Design review of the part built by this model. Coordinates are the model's own, in mm. A direction names the side the tool comes from. Coordinates: 2 decimals unless noted, no trailing zeros. Loops run counter-clockwise (first coordinate to the right, second up) from the corner with the lowest first, then second, coordinate; pieces in that order, holes last. Notation, with made-up numbers: (-39.5, 10.5) - (-2.5, 10.5) arc R21 cw to (-2.5, 30.5) - close; hole circle Ø8 at (-1.75, 71.25). An arc over 180 degrees is marked (long way). Answer in a Markdown table with one row per item. Add a question column.
(1) Clearance check with flat-ended pins moving along their axes: pin 1 (12 mm diameter, centred on y = 14, z = -4.5, fed in from -X); pin 2 (5 mm diameter, centred on y = 18, z = -3.5, fed in from +X); pin 3 (0.8 mm diameter, centred on x = -7, z = 0.5, fed in from +Y); pin 4 (3 mm diameter, centred on y = 14, z = -2, fed in from +X). State where each tip first meets the part, or that it passes through.
(2) We need section B-B, the plane x = 0. Write out the cut boundary in (y, z), plus the area to 3 significant figures.
(3) The part is to be moulded in two halves that separate along X. For faces 1 (the face through (3.3, 21.9, -0.1)), 2 (the face through (-8.321, 13.492, 0.845)), 3 (the face through (0.07, 37.76, 2.64)), say which applies: released by +X, released by -X, zero draft, split by the parting line, or undercut.
(4) We need section C-C, the plane y = 8.5. Write out the cut boundary in (x, z).
(5) We need section D-D, the plane y = 14.5. Write out the cut boundary in (x, z).
(6) For faces 4 (the face through (0, 37.9, 0)), 5 (the face through (0, 32, -1)), 6 (the face through (-1.08, 17.34, -4.88)), 7 (the face through (-7, 14.1, 0)), list the 3-axis set-ups (+Z, -Z, +X, -X, +Y, -Y) from which the entire face can be reached by the end or side of a thin tool; tool diameter is ignored.
(7) We need section A-A, the plane z = 0. Write out the cut boundary in (x, y).
(8) To check wall thickness, follow L1, parallel to Y at x = 0.5, z = 10; L2, parallel to X at y = 27, z = 0; L3, parallel to X at y = 22, z = -1. State the ranges of each line that lie inside material, in increasing order. Write a range as [from, to].
Autodesk Inventor part; units mm, degrees
ref_plane "YZ Plane" through (0, 0, 0) normal (1, 0, 0) x (0, 1, 0)
ref_plane "XZ Plane" through (0, 0, 0) normal (0, 1, 0) x (-1, 0, 0)
ref_plane "XY Plane" through (0, 0, 0) normal (0, 0, 1) x (1, 0, 0)
sketch "Sketch1" plane through (0, 0, 0) normal (0, 1, 0) x (-1, 0, 0)
  circle A0 centre (0, 0) radius 11.1
  dimension "d0" = 22.2
extrude "Extrusion1" add sketch "Sketch1" along normal blind 12.9
fillet "Fillet1" radius 0.3 1 edges at (11.1, 12.9, 0)
sketch "Sketch2" plane through (0, 12.9, 0) normal (0, 1, 0) x (1, 0, 0)
  circle A0 centre (0, 0) radius 5
  dimension "d4" = 10
extrude "Extrusion2" add sketch "Sketch2" along normal blind 9
sketch "Sketch3" plane through (0, 21.9, 0) normal (0, 1, 0) x (1, 0, 0)
  circle A0 centre (0, 0) radius 3
  dimension "d9" = 6
extrude "Extrusion3" add sketch "Sketch3" along normal blind 16
sketch "Sketch4" plane through (0, 12.9, 0) normal (0, 1, 0) x (1, 0, 0)
  circle A0 centre (-7.4, 0) radius 1.25
  circle A1 centre (0, 0) radius 3
  circle A2 centre (0, 0) radius 5
  dimension "d12" = 2.5
  dimension "d13" = 7.4
  dimension "d14" = 0
extrude "Extrusion4" add sketch "Sketch4" along normal blind 1.2 contours A0
chamfer "Chamfer1" distance 0.5 angle 45 1 edges at (-3, 37.9, 0)
sketch "Sketch5" plane through (0, 37.9, 0) normal (0, 1, 0) x (1, 0, 0)
  line L0 (-3.6948, 5.5128) -> (4.164, 5.5128)
  line L1 (4.164, 5.5128) -> (4.164, 1)
  line L2 (4.164, 1) -> (-3.6948, 1)
  line L3 (-3.6948, 1) -> (-3.6948, 5.5128)
  circle A0 centre (0, 0) radius 3
  dimension "d20" = 4
extrude "Extrusion5" cut sketch "Sketch5" against normal blind 12 contours L0 L1 L2 A0 L3 | A0 L2 picked at (0.6732, 1.4061)
properties part number "PotSensor"
Responses:
| question | item | result |
|---|---|---|
| 1 | pin 1 | stops at x = -11.1 |
| 1 | pin 2 | stops at x = 4.9 |
| 1 | pin 3 | stops at y = 14.1 |
| 1 | pin 4 | stops at x = 11.01 |
| 2 | outline | (0, -11.1) - (12.6, -11.1) arc R0.3 ccw to (12.9, -10.8) - (12.9, -5) - (21.9, -5) - (21.9, -3) - (25.9, -3) - (25.9, -1) - (37.9, -1) - (37.9, 2.5) - (37.4, 3) - (21.9, 3) - (21.9, 5) - (12.9, 5) - (12.9, 10.8) arc R0.3 ccw to (12.6, 11.1) - (0, 11.1) - close |
| 2 | area | 448 mm2 |
| 3 | face 1 | zero draft |
| 3 | face 2 | undercut |
| 3 | face 3 | split by the parting line |
| 4 | outline | circle Ø22.2 at (0, 0) |
| 5 | outline | circle Ø10 at (0, 0) |
| 6 | face 4 | +Z, -Z, +X, -X, +Y |
| 6 | face 5 | -Z, +X, -X, +Y |
| 6 | face 6 | +Y |
| 6 | face 7 | +Z, -Z, -X, +Y |
| 7 | outline | (-11.1, 0) - (11.1, 0) - (11.1, 12.6) arc R0.3 ccw to (10.8, 12.9) - (5, 12.9) - (5, 21.9) - (3, 21.9) - (3, 37.4) - (2.5, 37.9) - (-2.5, 37.9) - (-3, 37.4) - (-3, 21.9) - (-5, 21.9) - (-5, 12.9) - (-6.15, 12.9) - (-6.15, 14.1) - (-8.65, 14.1) - (-8.65, 12.9) - (-10.8, 12.9) arc R0.3 ccw to (-11.1, 12.6) - close |
| 8 | L1 | y = [0, 12.9] |
| 8 | L2 | x = [-3, 3] |
| 8 | L3 | x = [-2.83, 2.83] |
